Source: CAD feature listing. Evaluate the final solid. Frame: model axes, mm. A direction names the side the tool comes from. Coordinates: 2 decimals unless noted, no trailing zeros. Loops run counter-clockwise (first coordinate to the right, second up) from the corner with the lowest first, then second, coordinate; pieces in that order, holes last.
Item 1: Section query B-B, the plane y = -359.5. Return the cut outline in (x, z) (3 decimals), then the cut area to 3 significant figures.
Item 2: Reachability of faces 1 (the flat face through (193.662, -13, 33)), 2 (the flat face through (198.425, -13, 33)) from +Z, -Z, +X, -X, +Y, -Y: full face, straight path, thin tool, end or side. Return the list, or none.
Item 3: Line query: probe 1 along Z at (x, y) = (21.5, -322); probe 2 along X at (y, z) = (-317.5, 44.5); probe 3 along X at (y, z) = (-594.5, 1.5). Output: solid intervals per line, ascending.
Item 4: Pull-direction query (X, two-part tool) for faces 3 (the flat face through (-4.775, -13, 34)), 4 (the flat face through (0, -13, 31)), 5 (the flat face through (88.8, 914.4, -0.4)); classes: +X half, -X half, draft (parallel to the pull), parting line (faces both ways), or undercut.
Item 5: Section query A-A, the plane x = 72. Return the cut outline in (y, z).
```python
from build123d import *

# Parameters (mm, degrees)
F0_W     = 193.6623
F0_H     = 66.6623
F1_DEPTH = 914.4
F2_R     = 3.175


with BuildPart() as f1:
    # F0 (on Front) → F1 (new body, symmetric)
    with BuildSketch(Plane.XZ):
        Polygon((198.4248, -4.7752), (198.4248, 66.6623), (198.4248, 71.4248), (-4.7752, 71.4248), (-4.7752, -4.7752), align=None)
        with Locations((96.83115, 33.33115)):
            Rectangle(F0_W, F0_H, mode=Mode.SUBTRACT)
    extrude(amount=F1_DEPTH, both=True)

    # F2
    f2_edges = [f1.edges().sort_by_distance(p)[0] for p in [
        (-4.7752, 0, 71.4248),
        (0, 0, 66.6623),
        (-4.7752, 0, -4.7752),
        (198.4248, 0, -4.7752),
        (198.4248, 0, 71.4248),
        (193.6623, 0, 0),
        (193.6623, 0, 66.6623),
    ]]
    fillet(f2_edges, radius=F2_R)


solid = f1.part
```
Verdict:
1. outline: (-4.775, -1.6) arc R3.175 ccw to (-1.6, -4.775) - (195.25, -4.775) arc R3.175 ccw to (198.425, -1.6) - (198.425, 68.25) arc R3.175 ccw to (195.25, 71.425) - (-1.6, 71.425) arc R3.175 ccw to (-4.775, 68.25) - close; hole (0, 0) - (190.487, 0) arc R3.175 ccw to (193.662, 3.175) - (193.662, 63.487) arc R3.175 ccw to (190.487, 66.662) - (3.175, 66.662) arc R3.175 ccw to (0, 63.487) - close
1. area: 2,570 mm2
2. face 1: +Y, -Y
2. face 2: +Z, -Z, +X, +Y, -Y
3. probe 1: z = -4.78 to 0, 66.66 to 71.42
3. probe 2: x = -4.78 to 0, 193.66 to 198.42
3. probe 3: x = -4.78 to 0, 193.18 to 198.42
4. face 3: -X half
4. face 4: undercut
4. face 5: draft
5. outline: (-914.4, -4.78) - (914.4, -4.78) - (914.4, 0) - (-914.4, 0) - close; (-914.4, 66.66) - (914.4, 66.66) - (914.4, 71.42) - (-914.4, 71.42) - close
